Input: part model. Units: mm. Frame: model coordinates. Coordinates: 2 decimals unless noted, no trailing zeros. Write each loop counter-clockwise with the first axis right and the second up, starting at its lowest first coordinate (ties: lowest second). Pieces come first, ordered by that corner, then holes. Notation, with made-up numbers: (-2.5, 52) - (34.5, 52) arc R21 ccw to (34.5, 81) - close; hole circle Ø6 at (32, 43). An arc over 180 degrees is marked (long way). Use a Markdown table: item, result. Add a question column.
Q1. Pin query (flat end, axial travel): P1, Ø5, axis at y = 387.5, z = -41, coming from the +X side; P2, Ø4, axis at x = 0, y = 10.16, coming from the +Z side; P3, Ø6, axis at y = 369, z = -36.5, coming from the -X side; P4, Ø2, axis at x = -41.5, y = 56, coming from the -Z side. Return the tip coordinate at first contact, or that it passes through.
Q2. Section query A-A (y = 89). Return the cut outline in (x, z), then the cut area to 3 significant figures.
Q3. Material intervals for probe 1 along Y at (x, z) = (0, 55.75) (3 decimals); probe 2 along X at (y, z) = (170.5, 0); probe 3 along X at (y, z) = (45.5, -26), sorted ascending. Write a range as from..to.
Q4. Mould query, pull axis Y, two halves, no side actions, for faces 1 (the face through (-11.024, 2.976, -49.644)), 2 (the face through (40.301, 11.454, 35.888)), 3 (the face through (-35.888, 11.454, 40.301)), 4 (the face through (43, 498.475, -29)). Classes: released by +Y, released by -Y, zero draft, split by the parting line, or undercut.
Autodesk Inventor part; units mm, degrees
ref_plane "Work Plane1" through (57.15, 0, 0) normal (1, 0, 0) x (0, 1, 0)
ref_plane "XZ Plane" through (0, 0, 0) normal (0, 1, 0) x (-1, 0, 0)
ref_plane "XY Plane" through (0, 0, 0) normal (0, 0, 1) x (1, 0, 0)
sketch "Sketch1" plane through (0, 0, 0) normal (0, 1, 0) x (-1, 0, 0)
  circle A0 centre (0, 0) radius 57.15
  dimension "d0" = 114.3
extrude "Extrusion1" add sketch "Sketch1" along normal blind 498.475
sketch "Sketch2" plane through (0, 498.475, 0) normal (0, 1, 0) x (1, 0, 0)
  circle A0 centre (0, 0) radius 50.8
  dimension "d3" = 101.6
extrude "Extrusion2" cut sketch "Sketch2" against normal blind 609.6
ref_plane "Work Plane1" through (57.15, 0, 0) normal (1, 0, 0) x (0, 1, 0)
chamfer "Chamfer1" distance 3.175 angle 15 1 edges at (-50.8, 498.475, 0) measured on face at (-13.148, 166.1583, 49.069)
sketch "Sketch4" plane through (0, 0, 0) normal (0, 0, 1) x (1, 0, 0)
  circle A0 centre (0, 10.16) radius 3.3782
  point P0 (0, 0)
  dimension "d21" = 10.16
  dimension "d22" = 6.7564
extrude "Extrusion3" cut sketch "Sketch4" along normal through all
pattern_circular "Circular Pattern2" count 8 over 360 about axis through (0, -10, 0) along (0, 1, 0) of "Extrusion3"
chamfer "Chamfer2" distance 3.175 angle 15 1 edges at (-50.8, 0, 0) measured on face at (25.4, 165.1, 43.9941)
properties part number "Combustion Chamber" material "Aluminum 6061"
Values follow:
| question | item | result |
|---|---|---|
| 1 | P1 | x = 42.24 |
| 1 | P2 | through |
| 1 | P3 | x = -46.3 |
| 1 | P4 | z = -40.32 |
| 2 | outline | circle Ø114.3 at (0, 0); hole circle Ø101.6 at (0, 0) |
| 2 | area | 2,150 mm2 |
| 3 | probe 1 | 0..6.782, 13.538..498.475 |
| 3 | probe 2 | -57.15..-50.8, 50.8..57.15 |
| 3 | probe 3 | -50.89..-43.64, 43.64..50.89 |
| 4 | face 1 | released by -Y |
| 4 | face 2 | undercut |
| 4 | face 3 | undercut |
| 4 | face 4 | released by +Y |
